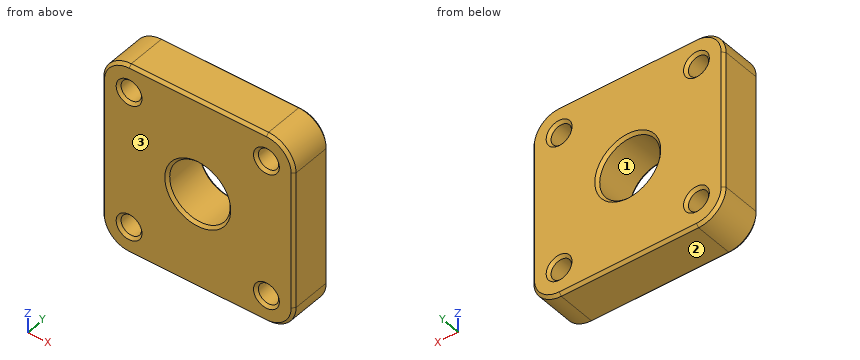
from build123d import *

# Parameters (mm, degrees)
SKETCH_1_W          = 70
SKETCH_1_H          = 70
EXTRUDE_1_DEPTH     = 16
SKETCH_2_R          = 11
SKETCH_2_R_2        = 3.7
CUT_EXTRUDE_1_DEPTH = 53.019227215
FILLET_1_R          = 10
CHAMFER_1_SIZE      = 1


with BuildPart() as part:
    # Эскиз1 → Бобышка-Вытянуть1 (new body)
    with BuildSketch(Plane(origin=(0, 0, 0), x_dir=(1, 0, 0), z_dir=(0, 1, 0))):
        Rectangle(SKETCH_1_W, SKETCH_1_H)
    extrude(amount=EXTRUDE_1_DEPTH)

    # Эскиз2 → Вырез-Вытянуть1 (cut, through all)
    with BuildSketch(Plane(origin=(0, 16, 0), x_dir=(1, 0, 0), z_dir=(0, 1, 0))):
        with Locations(Location((0, 0, 0), (0, 0, 270))):
            Circle(SKETCH_2_R)
        with Locations(Location((-25, 25, 0), (0, 0, 270))):
            Circle(SKETCH_2_R_2)
        with Locations(Location((25, 25, 0), (0, 0, 270))):
            Circle(SKETCH_2_R_2)
        with Locations(Location((25, -25, 0), (0, 0, 270))):
            Circle(SKETCH_2_R_2)
        with Locations(Location((-25, -25, 0), (0, 0, 270))):
            Circle(SKETCH_2_R_2)
    extrude(amount=-CUT_EXTRUDE_1_DEPTH, mode=Mode.SUBTRACT)

    # Скругление1
    fillet_1_edges = [part.edges().sort_by_distance(p)[0] for p in [
        (35, 8, 35),
        (-35, 8, 35),
        (-35, 8, -35),
        (35, 8, -35),
    ]]
    fillet(fillet_1_edges, radius=FILLET_1_R)

    # Фаска1
    chamfer_1_edges = [part.edges().sort_by_distance(p)[0] for p in [
        (-25, 0, 21.3),
        (-25, 16, 21.3),
        (25, 0, 21.3),
        (25, 16, 21.3),
        (25, 0, -28.7),
        (25, 16, -28.7),
        (-25, 0, -28.7),
        (-25, 16, -28.7),
        (0, 0, -11),
        (0, 16, -11),
        (0, 0, 35),
        (0, 16, 35),
        (35, 0, 0),
        (-35, 0, 0),
        (0, 0, -35),
        (32.071067812, 0, -32.071067812),
        (32.071067812, 0, 32.071067812),
        (-32.071067812, 0, -32.071067812),
        (-32.071067812, 0, 32.071067812),
        (-35, 16, 0),
        (35, 16, 0),
        (0, 16, -35),
        (32.071067812, 16, -32.071067812),
        (32.071067812, 16, 32.071067812),
        (-32.071067812, 16, -32.071067812),
        (-32.071067812, 16, 32.071067812),
    ]]
    chamfer(chamfer_1_edges, length=CHAMFER_1_SIZE)


solid = part.part
Input: part model. Units: mm. Frame: model coordinates. Face numbers are marked on the shaded views. Give positions to 0.01 mm unless a question says otherwise; leave off trailing zeros. Loops run counter-clockwise (first coordinate to the right, second up) from the corner with the lowest first, then second, coordinate; pieces in that order, holes last. Notation, with made-up numbers: (27.25, 18) - (51.25, 18) arc R18 ccw to (51.25, 39) - close; hole circle Ø7 at (-7.75, 85.25). An arc over 180 degrees is marked (long way). Use CSV: the item, a comma, the result in double quotes. Start each with the question number.
Item 1: Line query: line 1 (X direction, y = 10.25, z = 25); line 2 (X direction, y = 5.25, z = 0); line 3 (Z direction, x = 23, y = 13.5). Output: solid intervals per line, ascending.
Item 2: Section B-B on y = 5.25. Return loops of the section in (x, z), then the cut area to 3 significant figures.
Item 3: Section A-A on x = 0. Return loops of the section in (y, z), then the cut area to 3 significant figures.
Item 4: Contact query for flat-ended pins moving along their axis: P1, Ø8.5, axis at x = -25, z = -25, coming from the +Y side; P2, Ø8.5, axis at x = 25, z = 25, coming from the -Y side. Output: stop coordinate, or through.
Item 5: Mould query, pull axis Z, two halves, no side actions, for the marked faces 1, 2 and 3. Classes: pulls with the +Z half, pulls with the -Z half, needs draft (parallel to the pull), parting line crosses it, or undercut.
Item 6: Section C-C on x = -23.5. State how many separate pieces and enclosed holes the cut face has, then the cut area to 3 significant figures.
Ans:
1,line 1,"x = -35 to -28.7, -21.3 to 21.3, 28.7 to 35"
1,line 2,"x = -35 to -11, 11 to 35"
1,line 3,"z = -35 to -28.11, -21.89 to 21.89, 28.11 to 35"
2,outline,"(-35, -25) arc R10 ccw to (-25, -35) - (25, -35) arc R10 ccw to (35, -25) - (35, 25) arc R10 ccw to (25, 35) - (-25, 35) arc R10 ccw to (-35, 25) - close; hole circle Ø7.4 at (-25, -25); hole circle Ø7.4 at (-25, 25); hole circle Ø22 at (0, 0); hole circle Ø7.4 at (25, -25); hole circle Ø7.4 at (25, 25)"
2,area,"4,260 mm2"
3,outline,"(0, -34) - (1, -35) - (15, -35) - (16, -34) - (16, -12) - (15, -11) - (1, -11) - (0, -12) - close; (0, 12) - (1, 11) - (15, 11) - (16, 12) - (16, 34) - (15, 35) - (1, 35) - (0, 34) - close"
3,area,"764 mm2"
4,P1,"stops at y = 15.55"
4,P2,"stops at y = 0.45"
5,face 1,"undercut"
5,face 2,"pulls with the -Z half"
5,face 3,"needs draft"
6,separate pieces,"3"
6,enclosed holes,"0"
6,area,"897 mm2"
